The model under review builds one solid part; all positions refer to its coordinate system, in mm. Face numbers are marked on the shaded views. A direction names the side the tool comes from. Coordinates: 2 decimals unless noted, no trailing zeros. Write each loop counter-clockwise with the first axis right and the second up, starting at its lowest first coordinate (ties: lowest second). Pieces come first, ordered by that corner, then holes.
1) For P1, Ø4, axis at x = 30, z = 14, coming from the +Y side; P2, Ø3, axis at y = 33, z = 18, coming from the +X side; P3, Ø2, axis at x = 17.5, z = 19, coming from the +Y side, all flat-tipped, find the tip position at first contact; note any pin that passes through.
2) Mouldability with a two-part tool opening along Z and no side actions: class the marked faces 1, 2 and 3 as released by +Z, released by -Z, zero draft, split by the parting line, or undercut.
3) For line 1 (Z direction, x = 22.5, y = 27); line 2 (Y direction, x = 7.5, z = 18); line 3 (Z direction, x = 23.5, y = 26), list the stretches that pass through material, from the lowest coordinate up.
4) Machinability: for the marked faces 4, 5, 6 and 7, which of the approach directions +Z, -Z, +X, -X, +Y, -Y give a long, thin tool a straight path to every point of the face, cutting with its end or side? Answer none if there is none.
5) Add section A-A, the plane y = 27.5. State the section outline as (x, z) points.
from build123d import *

# Parameters (mm, degrees)
PAD_DEPTH       = 30
POCKET_DEPTH    = 42.067391
FILLET_R        = 8.5
SKETCH002_R     = 3.2
POCKET001_DEPTH = 56.997477
SKETCH003_R     = 5.5
POCKET002_DEPTH = 46.997477
FILLET001_R     = 2
CHAMFER_SIZE    = 1


with BuildPart() as part:
    # Sketch → Pad (new body)
    with BuildSketch(Plane.XY):
        with BuildLine():
            Line((33.560053, 32.310668), (5.525773, 13.017904))
            Line((5.525773, 13.017904), (9.271839, 3.746066))
            Line((9.271839, 3.746066), (0, 0))
            Line((0, 0), (-6.986015, 17.290994))
            Line((-6.986015, 17.290994), (15.957042, 50.057076))
            ThreePointArc((33.560053, 32.310668), (35.376884, 51.716409), (15.957042, 50.057076))
        make_face()
    extrude(amount=PAD_DEPTH)

    # Sketch001 (on Face1 of Pad) → Pocket (cut, through all)
    with BuildSketch(Plane(origin=(-4.303566, 6.253504, 0), x_dir=(0.823779, 0.566912, 0), z_dir=(0.566912, -0.823779, 0))):
        Polygon((25.963349, 4), (14.963349, 15), (25.963349, 26), (35.963349, 26), (35.963349, 4), align=None)
    extrude(amount=-POCKET_DEPTH, mode=Mode.SUBTRACT)

    # Fillet
    fillet_edges = [part.edges().sort_by_distance(p)[0] for p in [
        (12.55333, 45.196071, 15),
        (25.322268, 26.64155, 15),
    ]]
    fillet(fillet_edges, radius=FILLET_R)

    # Sketch002 (on Face15 of Fillet) → Pocket001 (cut, through all)
    with BuildSketch(Plane(origin=(0, 0, 0), x_dir=(0.374607, -0.927184, 0), z_dir=(-0.927184, -0.374607, 0))):
        with Locations((-11, 15)):
            Circle(SKETCH002_R)
    extrude(amount=-POCKET001_DEPTH, mode=Mode.SUBTRACT)

    # Sketch003 (on Face5 of Pocket001) → Pocket002 (cut, through all)
    with BuildSketch(Plane(origin=(9.271839, 3.746066, 0), x_dir=(-0.374607, 0.927184, 0), z_dir=(0.927184, 0.374607, 0))):
        with Locations((11, 15)):
            Circle(SKETCH003_R)
    extrude(amount=POCKET002_DEPTH, mode=Mode.SUBTRACT)

    # Fillet001
    fillet001_edges = [part.edges().sort_by_distance(p)[0] for p in [
        (9.271839, 3.746066, 15),
        (0, 0, 15),
    ]]
    fillet(fillet001_edges, radius=FILLET001_R)

    # Chamfer
    chamfer_edges = [part.edges().sort_by_distance(p)[0] for p in [
        (7.024199, 9.309169, 0),
        (8.509267, 4.069758, 0),
        (19.542913, 22.664286, 0),
        (4.635919, 1.873033, 0),
        (35.376884, 51.716409, 0),
        (0.323692, 0.762571, 0),
        (4.485514, 33.674035, 0),
        (-3.867614, 9.572681, 0),
        (7.024199, 9.309169, 30),
        (8.509267, 4.069758, 30),
        (19.542913, 22.664286, 30),
        (4.635919, 1.873033, 30),
        (35.376884, 51.716409, 30),
        (0.323692, 0.762571, 30),
        (4.485514, 33.674035, 30),
        (-3.867614, 9.572681, 30),
    ]]
    chamfer(chamfer_edges, length=CHAMFER_SIZE)


solid = part.part
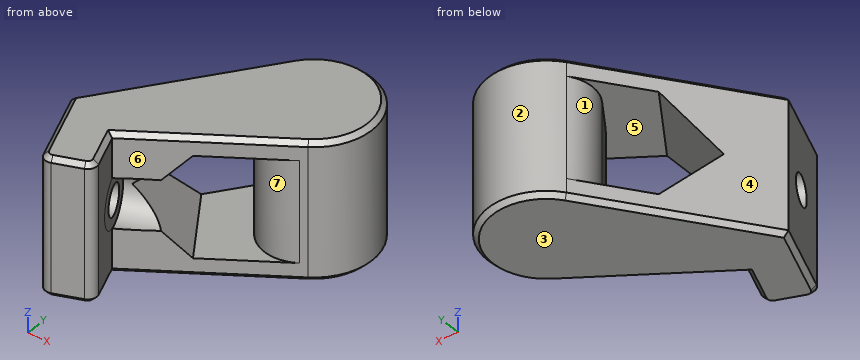
Geometry results:
1. P1: stops at y = 55.37
1. P2: stops at x = 36
1. P3: stops at y = 52.75
2. face 1: undercut
2. face 2: zero draft
2. face 3: released by -Z
3. line 1: z = 0 to 4, 26 to 30
3. line 2: y = 3.03 to 8.13, 19.87 to 20.79
3. line 3: z = 0.5 to 4, 26 to 29.5
4. face 4: +Z, -Z, -X, +Y
4. face 5: none
4. face 6: +Z, -Z, +X
4. face 7: -Y
5. outline: (0.16, 1) - (1.38, 0) - (24.81, 0) - (26.57, 1) - (26.57, 4) - (12.59, 4) - (0.16, 14.24) - close; (0.16, 15.76) - (12.59, 26) - (26.57, 26) - (26.57, 29) - (24.81, 30) - (1.38, 30) - (0.16, 29) - close
